Build history of the part. All positions in model axes, mm. Face numbers are marked on the shaded views. A direction names the side the tool comes from. Round coordinates to 2 decimals unless told otherwise and drop trailing zeros. Order: outer loops, then holes, each group sorted by start corner. A loop starts at its lowest first (then second) coordinate and runs counter-clockwise, first axis right, second up. Notation, with made-up numbers: (73.5, 12.5) -> (80.5, 12.5) arc R9 cw to (80.5, 25.5) -> close; hole circle Ø4 at (45, 33.5). An arc over 180 degrees is marked (long way). Answer as a JSON object with one key per item and string values.
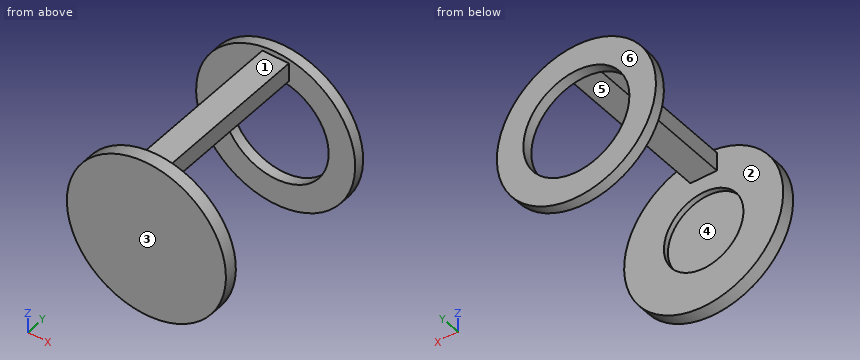
from build123d import *

# Parameters (mm, degrees)
SKETCH1_R           = 38.1
SKETCH1_R_2         = 25.4
BOSS_EXTRUDE1_DEPTH = 5.08
SKETCH4_W           = 12.7
SKETCH4_H           = 8.89
BOSS_EXTRUDE3_DEPTH = 76.2
SKETCH5_R           = 38.1
BOSS_EXTRUDE4_DEPTH = 6.35
SKETCH6_R           = 19.05
CUT_EXTRUDE1_DEPTH  = 2.54


with BuildPart() as part:
    # Sketch1 → Boss-Extrude1 (new body)
    with BuildSketch(Plane(origin=(0, 0, 0), x_dir=(1, 0, 0), z_dir=(0, 1, 0))):
        with Locations(Location((0, 0, 0), (0, 0, 270))):  # turned: the seam where the file's is
            Circle(SKETCH1_R)
        with Locations(Location((0, 0, 0), (0, 0, 270))):  # turned: the seam where the file's is
            Circle(SKETCH1_R_2, mode=Mode.SUBTRACT)
    extrude(amount=BOSS_EXTRUDE1_DEPTH)

    # Sketch4 → Boss-Extrude3 (add)
    with BuildSketch(Plane.XZ):
        with Locations((0, 31.115)):
            Rectangle(SKETCH4_W, SKETCH4_H)
    extrude(amount=BOSS_EXTRUDE3_DEPTH)

    # Sketch5 → Boss-Extrude4 (add)
    with BuildSketch(Plane.XZ.offset(76.2)):
        with Locations(Location((0, 0, 0), (0, 0, 90))):  # turned: the seam where the file's is
            Circle(SKETCH5_R)
    extrude(amount=BOSS_EXTRUDE4_DEPTH)

    # Sketch6 → Cut-Extrude1 (cut)
    with BuildSketch(Plane(origin=(0, -76.2, 0), x_dir=(1, 0, 0), z_dir=(0, 1, 0))):
        with Locations(Location((0, 0, 0), (0, 0, 270))):  # turned: the seam where the file's is
            Circle(SKETCH6_R)
    extrude(amount=-CUT_EXTRUDE1_DEPTH, mode=Mode.SUBTRACT)


solid = part.part
1) Cut at C-C, the plane x = 22.5. Give the cut face in (y, z).
Checked values:
{"outline": "(-82.55, -30.75) -> (-76.2, -30.75) -> (-76.2, 30.75) -> (-82.55, 30.75) -> close; (0, -30.75) -> (5.08, -30.75) -> (5.08, -11.79) -> (0, -11.79) -> close; (0, 11.79) -> (5.08, 11.79) -> (5.08, 30.75) -> (0, 30.75) -> close"}
2) Which spindle directions (+Z, -Z, +X, -X, +Y, -Y) get a long thin tool onto all of the face, cutting with end or side? Do the marked faces 5 and 6. Say none if no direction does.
Checked values:
{"face 5": "-Z, +X, -X", "face 6": "+Z, -Z, +X, -X, +Y"}
3) Flat gauge pins, fed straight in: pin 1 Ø4.5 at (y, z) = (-38.5, 29.5) entering from +X; pin 2 Ø23 at (x, z) = (-8, -5.5) entering from +Y; pin 3 Ø2.5 at (y, z) = (-56.5, 31.5) entering from -X; pin 4 Ø6 at (x, y) = (13, -70.5) entering from +Z. Where does each tip first touch, or does it go through?
Checked values:
{"pin 1": "stops at x = 6.35", "pin 2": "stops at y = -76.2", "pin 3": "stops at x = -6.35", "pin 4": "passes through"}
4) Cut at A-A, the plane z = 0. Give the cut face in (x, y).
Checked values:
{"outline": "(-38.1, -82.55) -> (38.1, -82.55) -> (38.1, -76.2) -> (19.05, -76.2) -> (19.05, -78.74) -> (-19.05, -78.74) -> (-19.05, -76.2) -> (-38.1, -76.2) -> close; (-38.1, 0) -> (-25.4, 0) -> (-25.4, 5.08) -> (-38.1, 5.08) -> close; (25.4, 0) -> (38.1, 0) -> (38.1, 5.08) -> (25.4, 5.08) -> close"}
5) Pull direction Y, two halves, no side cores. Call the marked faces 1, 2, 3 and 4: pulls with the +Y half, pulls with the -Y half, needs draft (parallel to the pull), parting line crosses it, or undercut.
Checked values:
{"face 1": "undercut", "face 2": "undercut", "face 3": "pulls with the -Y half", "face 4": "pulls with the +Y half"}
6) Cut at B-B, the plane x = 0. Give the cut face in (y, z), plus the area to 3 significant figures.
Checked values:
{"outline": "(-82.55, -38.1) -> (-76.2, -38.1) -> (-76.2, -19.05) -> (-78.74, -19.05) -> (-78.74, 19.05) -> (-76.2, 19.05) -> (-76.2, 26.67) -> (0, 26.67) -> (0, 25.4) -> (5.08, 25.4) -> (5.08, 38.1) -> (0, 38.1) -> (0, 35.56) -> (-76.2, 35.56) -> (-76.2, 38.1) -> (-82.55, 38.1) -> close; (0, -38.1) -> (5.08, -38.1) -> (5.08, -25.4) -> (0, -25.4) -> close", "area": "1,190 mm²"}
7) Probe L1, parallel to Y at x = -25, z = -19; L2, parallel to X at y = -77.2, z = 0; L3, parallel to Y at x = 7.5, z = 7. List the from-to ranges inside material, lowest first. Write a range as from..to.
Checked values:
{"L1": "y = -82.55..-76.2, 0..5.08", "L2": "x = -38.1..-19.05, 19.05..38.1", "L3": "y = -82.55..-78.74"}
8) Cut at D-D, the plane z = -15. Give the cut face in (x, y).
Checked values:
{"outline": "(-35.02, -82.55) -> (35.02, -82.55) -> (35.02, -76.2) -> (11.74, -76.2) -> (11.74, -78.74) -> (-11.74, -78.74) -> (-11.74, -76.2) -> (-35.02, -76.2) -> close; (-35.02, 0) -> (-20.5, 0) -> (-20.5, 5.08) -> (-35.02, 5.08) -> close; (20.5, 0) -> (35.02, 0) -> (35.02, 5.08) -> (20.5, 5.08) -> close"}
